from build123d import *

# Parameters (mm, degrees)
SKETCH_1_W                         = 321
SKETCH_1_H                         = 60
SM_BASE_FLANGE_1_DEPTH             = 1.5
SM_EDGE_FLANGE_1_STRIP_W           = 7
SM_EDGE_FLANGE_1_STRIP_H           = 1.5
SM_EDGE_FLANGE_1_STRIP_CUT_DEPTH   = 321
SM_EDGE_FLANGE_1_STRIP_2_W         = 7
SM_EDGE_FLANGE_1_STRIP_2_H         = 1.5
SM_EDGE_FLANGE_1_STRIP_CUT_2_DEPTH = 321
SM_EDGE_FLANGE_1_DEPTH             = 321
SM_EDGE_FLANGE_1_BEND_DEPTH        = 321
SM_EDGE_FLANGE_2_STRIP_W           = 7
SM_EDGE_FLANGE_2_STRIP_H           = 1.5
SM_EDGE_FLANGE_2_STRIP_CUT_DEPTH   = 321
SM_EDGE_FLANGE_2_STRIP_2_W         = 7
SM_EDGE_FLANGE_2_STRIP_2_H         = 1.5
SM_EDGE_FLANGE_2_STRIP_CUT_2_DEPTH = 321
SM_EDGE_FLANGE_2_DEPTH             = 321
SM_EDGE_FLANGE_2_BEND_DEPTH        = 321
CUT_EXTRUDE_2_DEPTH                = 174.385408844
CUT_EXTRUDE_3_DEPTH                = 57
CUT_EXTRUDE_3_DEPTH_BACK           = 10
SKETCH_20_W                        = 341.087454661
SKETCH_20_H                        = 74.910603127


# Sheet-metal steps are written as plain solids
with BuildPart() as part:
    # Sketch 1 → 基体-法兰1 (new body)
    with BuildSketch(Plane.XY):
        Rectangle(SKETCH_1_W, SKETCH_1_H)
    extrude(amount=-SM_BASE_FLANGE_1_DEPTH)

    # 边线-法兰1 strip (across the edge) → 边线-法兰1 strip cut (cut)
    with BuildSketch(Plane(origin=(160.5, 30, 0), x_dir=(0, -1, 0), z_dir=(-1, 0, 0))):
        with Locations((-1.5, -0.75)):
            Rectangle(SM_EDGE_FLANGE_1_STRIP_W, SM_EDGE_FLANGE_1_STRIP_H)
    extrude(amount=SM_EDGE_FLANGE_1_STRIP_CUT_DEPTH, mode=Mode.SUBTRACT)

    # 边线-法兰1 strip 2 (across the edge) → 边线-法兰1 strip cut 2 (cut)
    with BuildSketch(Plane(origin=(-160.5, -30, 0), x_dir=(0, 1, 0), z_dir=(1, 0, 0))):
        with Locations((-1.5, -0.75)):
            Rectangle(SM_EDGE_FLANGE_1_STRIP_2_W, SM_EDGE_FLANGE_1_STRIP_2_H)
    extrude(amount=SM_EDGE_FLANGE_1_STRIP_CUT_2_DEPTH, mode=Mode.SUBTRACT)

    # 边线-法兰1 section (across the edge) → 边线-法兰1 (add)
    with BuildSketch(Plane(origin=(160.5, 30, 0), x_dir=(0, -1, 0), z_dir=(-1, 0, 0))):
        with BuildLine():
            Line((0, 0.5), (0, 26.5))
            Line((0, 26.5), (1.5, 26.5))
            Line((1.5, 26.5), (1.5, 0.5))
            ThreePointArc((1.5, 0.5), (1.646446609, 0.146446609), (2, 0))
            Line((2, 0), (2, -1.5))
            ThreePointArc((2, -1.5), (0.585786438, -0.914213562), (0, 0.5))
        make_face()
    extrude(amount=SM_EDGE_FLANGE_1_DEPTH)

    # 边线-法兰1 section 2 (across the edge) → 边线-法兰1 bend (add)
    with BuildSketch(Plane(origin=(-160.5, -30, 0), x_dir=(0, 1, 0), z_dir=(1, 0, 0))):
        with BuildLine():
            Line((0, 0.5), (0, 26.5))
            Line((0, 26.5), (1.5, 26.5))
            Line((1.5, 26.5), (1.5, 0.5))
            ThreePointArc((1.5, 0.5), (1.646446609, 0.146446609), (2, 0))
            Line((2, 0), (2, -1.5))
            ThreePointArc((2, -1.5), (0.585786438, -0.914213562), (0, 0.5))
        make_face()
    extrude(amount=SM_EDGE_FLANGE_1_BEND_DEPTH)

    # 边线-法兰2 strip (across the edge) → 边线-法兰2 strip cut (cut)
    with BuildSketch(Plane(origin=(160.5, 28.5, 26.5), x_dir=(0, 0, -1), z_dir=(-1, 0, 0))):
        with Locations((-1.5, -0.75)):
            Rectangle(SM_EDGE_FLANGE_2_STRIP_W, SM_EDGE_FLANGE_2_STRIP_H)
    extrude(amount=SM_EDGE_FLANGE_2_STRIP_CUT_DEPTH, mode=Mode.SUBTRACT)

    # 边线-法兰2 strip 2 (across the edge) → 边线-法兰2 strip cut 2 (cut)
    with BuildSketch(Plane(origin=(-160.5, -28.5, 26.5), x_dir=(0, 0, -1), z_dir=(1, 0, 0))):
        with Locations((-1.5, -0.75)):
            Rectangle(SM_EDGE_FLANGE_2_STRIP_2_W, SM_EDGE_FLANGE_2_STRIP_2_H)
    extrude(amount=SM_EDGE_FLANGE_2_STRIP_CUT_2_DEPTH, mode=Mode.SUBTRACT)

    # 边线-法兰2 section (across the edge) → 边线-法兰2 (add)
    with BuildSketch(Plane(origin=(160.5, 28.5, 26.5), x_dir=(0, 0, -1), z_dir=(-1, 0, 0))):
        with BuildLine():
            Line((0, 0.5), (0, 8.5))
            Line((0, 8.5), (1.5, 8.5))
            Line((1.5, 8.5), (1.5, 0.5))
            ThreePointArc((1.5, 0.5), (1.646446609, 0.146446609), (2, 0))
            Line((2, 0), (2, -1.5))
            ThreePointArc((2, -1.5), (0.585786438, -0.914213562), (0, 0.5))
        make_face()
    extrude(amount=SM_EDGE_FLANGE_2_DEPTH)

    # 边线-法兰2 section 2 (across the edge) → 边线-法兰2 bend (add)
    with BuildSketch(Plane(origin=(-160.5, -28.5, 26.5), x_dir=(0, 0, -1), z_dir=(1, 0, 0))):
        with BuildLine():
            Line((0, 0.5), (0, 8.5))
            Line((0, 8.5), (1.5, 8.5))
            Line((1.5, 8.5), (1.5, 0.5))
            ThreePointArc((1.5, 0.5), (1.646446609, 0.146446609), (2, 0))
            Line((2, 0), (2, -1.5))
            ThreePointArc((2, -1.5), (0.585786438, -0.914213562), (0, 0.5))
        make_face()
    extrude(amount=SM_EDGE_FLANGE_2_BEND_DEPTH)

    # 草图19 → 切除-拉伸2 (cut, through all)
    with BuildSketch(Plane(origin=(0, 30, 0), x_dir=(1, 0, 0), z_dir=(0, 1, 0))):
        with BuildLine():
            Line((-132, -5), (-18, -5))
            ThreePointArc((-18, -5), (-15.878679656, -5.878679656), (-15, -8))
            Line((-15, -8), (-15, -17))
            ThreePointArc((-15, -17), (-15.878679656, -19.121320344), (-18, -20))
            Line((-18, -20), (-132, -20))
            ThreePointArc((-132, -20), (-134.121320344, -19.121320344), (-135, -17))
            Line((-135, -17), (-135, -8))
            ThreePointArc((-135, -8), (-134.121320344, -5.878679656), (-132, -5))
        make_face()
    cut_extrude_2 = extrude(amount=-CUT_EXTRUDE_2_DEPTH, mode=Mode.SUBTRACT)

    # 镜向1: 切除-拉伸2 across plane
    add(cut_extrude_2.mirror(Plane(origin=(0, 0, 0), x_dir=(0, 0, 1), z_dir=(1, 0, 0))), mode=Mode.SUBTRACT)

    # 草图20 → 切除-拉伸3 (cut, two sides: drawn at the far end of the back side and taken through both)
    with BuildSketch(Plane.XY.offset(-CUT_EXTRUDE_3_DEPTH_BACK)):
        with Locations((-10.043727331, -17.455301564)):
            Rectangle(SKETCH_20_W, SKETCH_20_H)
    extrude(amount=CUT_EXTRUDE_3_DEPTH + CUT_EXTRUDE_3_DEPTH_BACK, mode=Mode.SUBTRACT)


solid = part.part
The model under review builds one solid part; all positions refer to its coordinate system, in mm. A direction names the side the tool comes from. Round coordinates to 2 decimals unless told otherwise and drop trailing zeros. Write each loop counter-clockwise with the first axis right and the second up, starting at its lowest first coordinate (ties: lowest second). Pieces come first, ordered by that corner, then holes. Notation, with made-up numbers: M 89,54.25 L 134,54.25 A9 ccw 134,58.25 Z; hole C 8.25,30.5 d6. An arc over 180 degrees is marked long. Answer as CSV lines item,"result". Start each with the question number.
Q1. Wall thickness on line 1 along Z through (x, y) = (-75, 25.5); line 2 along X through (y, z) = (29.5, 18.25); line 3 along Y through (x, z) = (65.5, 23.25): over which ranges is each line inside the solid? List them lowest first.
Q2. Tool access review of faces 4 (the face through (2, 28.5, 13)), 5 (the face through (2, 24, 26.5)): name each direction out of +Z, -Z, +X, -X, +Y, -Y from which nothing blocks a thin tool from reaching the whole face with its end or side.
Q3. Consider section C-C, the plane y = 23.5. Give the boundary of the cut face in (x, z).
Q4. Clearance check with flat-ended pins moving along their axes: P1, Ø5, axis at y = 24, z = 8.5, coming from the +X side; P2, Ø3, axis at x = -69, z = 19, coming from the -Y side; P3, Ø1.6, axis at x = 68.5, y = 29.5, coming from the -Z side; P4, Ø1.2, axis at x = 98, y = 29.5, coming from the +Z side. State where each tip first meets the part, or that it passes through.
Q5. Consider section D-D, the plane x = 11. Give the boundary of the cut face in (y, z), then the cut area to 3 significant figures.
Q6. Consider section B-B, the plane x = 110.5. Give the boundary of the cut face in (y, z), then the cut area to 3 significant figures.
Q7. The part is to be moulded in two halves that separate along Z. For faces 1 (the face through (-2, 24, -1.5)), 2 (the face through (160.5, 29, 10)), 3 (the face through (2, 24, 25)), say which applies: +Z half, -Z half, draft (parallel to the pull), parting line (faces both ways), or undercut.
Q8. Consider section A-A, the plane z = 13.25. Give the boundary of the cut face in (x, y), then the cut area to 4 significant figures.
Result set:
1,line 1,"z = -1.5 to 0, 25 to 26.5"
1,line 2,"x = -160.5 to -134.73, -15.27 to 15.27, 134.73 to 160.5"
1,line 3,"y = 28.5 to 30"
2,face 4,"+X, -X, -Y"
2,face 5,"+Z, +X, -X, +Y, -Y"
3,outline,"M -160.5,-1.5 L 160.5,-1.5 L 160.5,0 L -160.5,0 Z; M -160.5,25 L 160.5,25 L 160.5,26.5 L -160.5,26.5 Z"
4,P1,"passes through"
4,P2,"stops at y = 28.5"
4,P3,"stops at z = -1.37"
4,P4,"stops at z = 26.29"
5,outline,"M 20,-1.5 L 28,-1.5 A2 ccw 30,0.5 L 30,24.5 A2 ccw 28,26.5 L 20,26.5 L 20,25 L 28,25 A0.5 cw 28.5,24.5 L 28.5,0.5 A0.5 cw 28,0 L 20,0 Z"
5,area,"65.9 mm²"
6,outline,"M 20,-1.5 L 28,-1.5 A2 ccw 30,0.5 L 30,5 L 28.5,5 L 28.5,0.5 A0.5 cw 28,0 L 20,0 Z; M 20,25 L 28,25 A0.5 cw 28.5,24.5 L 28.5,20 L 30,20 L 30,24.5 A2 ccw 28,26.5 L 20,26.5 Z"
6,area,"43.4 mm²"
7,face 1,"-Z half"
7,face 2,"draft"
7,face 3,"undercut"
8,outline,"M -160.5,28.5 L -135,28.5 L -135,30 L -160.5,30 Z; M -15,28.5 L 15,28.5 L 15,30 L -15,30 Z; M 135,28.5 L 160.5,28.5 L 160.5,30 L 135,30 Z"
8,area,"121.5 mm²"
